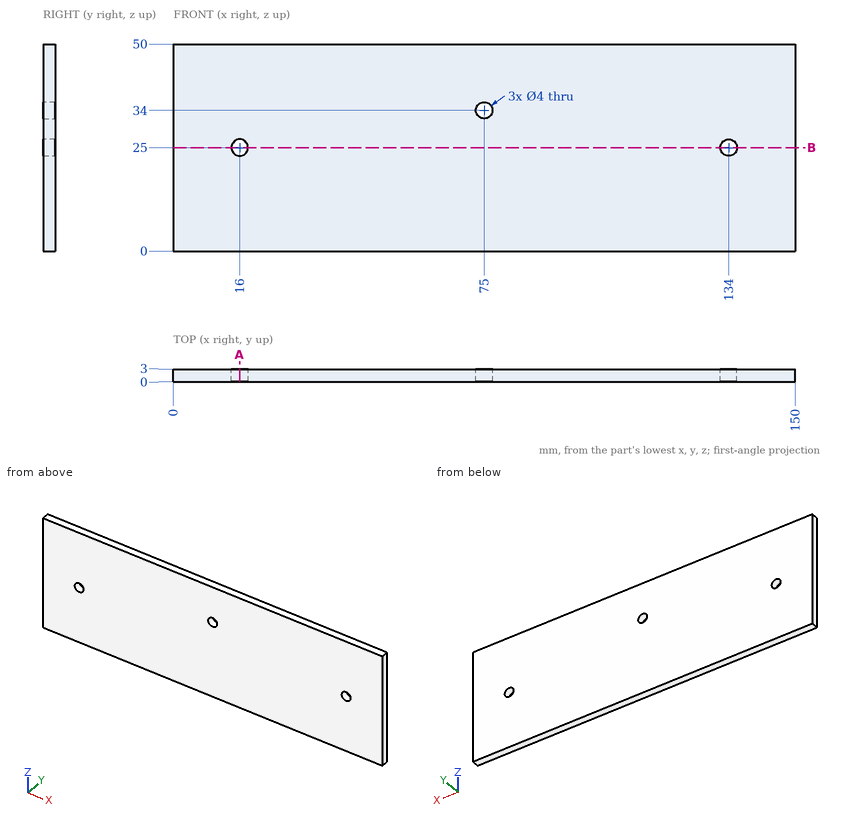
Input: dimensioned drawing with shaded views. Units: mm. Origin: part minimum x, y, z. Give positions to 0.01 mm unless a question says otherwise; leave off trailing zeros. Order: outer loops, then holes, each group sorted by start corner. A loop starts at its lowest first (then second) coordinate and runs counter-clockwise, first axis right, second up. Notation, with made-up numbers: (-3.5, 60) -> (24.5, 60) arc R19 ccw to (24.5, 89) -> close; hole circle Ø11 at (52, 1). An arc over 180 degrees is marked (long way). Write item = value, one per line.
Item 1: Contact query for a flat-ended pin moving along its axis: pin 1 (4 mm diameter, centred on x = 22.5, z = 12.5, fed in from -Y). Output: stop coordinate, or through.
Check result:
pin_1 = 0
Item 2: Section query A-A (x = 16). Output: boundary loops of the cut face in (y, z), then the cut area to 3 significant figures.
Check result:
outline = (0, 0) -> (3, 0) -> (3, 23) -> (0, 23) -> close; (0, 27) -> (3, 27) -> (3, 50) -> (0, 50) -> close
area = 138 mm²
Item 3: Section query B-B (z = 25). Output: boundary loops of the cut face in (x, y).
Check result:
outline = (0, 0) -> (14, 0) -> (14, 3) -> (0, 3) -> close; (18, 0) -> (132, 0) -> (132, 3) -> (18, 3) -> close; (136, 0) -> (150, 0) -> (150, 3) -> (136, 3) -> close
Item 4: Ray query, probe 1 along X at (y, z) = (1.45, 25); probe 2 along Z at (x, y) = (134, 1.95); probe 3 along X at (y, z) = (1.2, 34). Return the intervals inside material, ascending.
Check result:
probe_1 = 0 to 14, 18 to 132, 136 to 150
probe_2 = 0 to 23, 27 to 50
probe_3 = 0 to 73, 77 to 150
